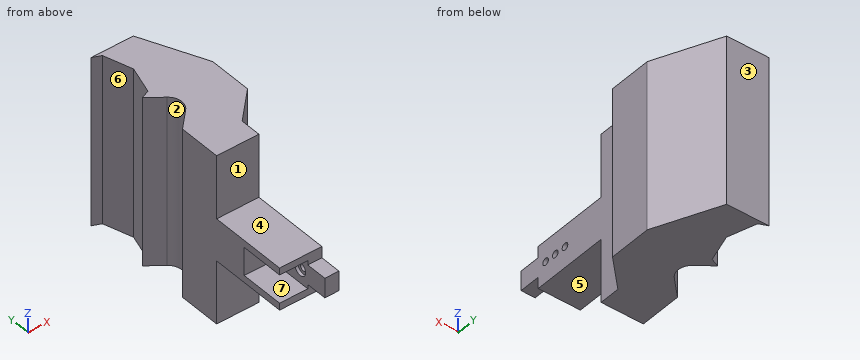
Autodesk Inventor part; units mm, degrees
ref_plane "Work Plane1" through (0, 0, -15) normal (0, 0, 1) x (1, 0, 0)
ref_plane "YZ Plane" through (0, 0, 0) normal (1, 0, 0) x (0, 1, 0)
ref_plane "XZ Plane" through (0, 0, 0) normal (0, 1, 0) x (-1, 0, 0)
sketch "Sketch1" plane through (0, 0, 0) normal (0, 0, 1) x (1, 0, 0)
  line L0 (0, 0) -> (25, 0)
  line L1 (25, 0) -> (25, 40)
  line L2 (25, 40) -> (0, 40)
  line L3 (0, 40) -> (0, 0)
  dimension "d1" = 25
  dimension "d2" = 40
  dimension "d3" = 25
extrude "Extrusion1" add sketch "Sketch1" against normal blind 30
sketch "Sketch2" plane through (25, 0, 0) normal (1, 0, 0) x (0, 0, -1)
  line L0 (0, 0) -> (30, 0)
  circle A0 centre (15, 6.56) radius 2.46
extrude "Extrusion2" cut sketch "Sketch2" against normal blind 30
sketch "Sketch3" plane through (0, 0, 0) normal (-1, 0, 0) x (0, 0, 1)
  line L0 (0, 0) -> (-30, 0)
  line L1 (-25.05, 0) -> (-4.95, 0)
  line L2 (-4.95, 0) -> (-4.95, 33.12)
  line L3 (-4.95, 33.12) -> (-25.05, 33.12)
  line L4 (-25.05, 33.12) -> (-25.05, 0)
  dimension "d11" = 20.1
extrude "Extrusion3" cut sketch "Sketch3" against normal blind 20
sketch "Sketch4" plane through (0, 0, 0) normal (0, -1, 0) x (1, 0, 0)
  line L0 (20, -4.95) -> (20, -25.05)
  line L1 (20, -15) -> (25, -15)
  line L2 (25, 0) -> (25, -30)
  line L3 (20, -8.025) -> (25, -8.025)
  line L4 (25, -8.025) -> (25, -21.975)
  line L5 (25, -21.975) -> (20, -21.975)
  line L6 (20, -21.975) -> (20, -8.025)
  line L7 (20, -8.025) -> (25, -21.975) construction
  line L8 (25, -8.025) -> (20, -21.975) construction
  line L9 (25, -12.54) -> (25, -17.46)
  point P0 (0, 0)
  point P1 (22.5, -15)
  dimension "d14" = 13.95
extrude "Extrusion4" add sketch "Sketch4" along normal blind 15
sketch "Sketch5" plane through (20, 0, 0) normal (-1, 0, 0) x (0, 0, 1)
  circle A0 centre (-15, 6.56) radius 2.46
  circle A1 centre (-15, 6.56) radius 4.7025
  circle A2 centre (-15, 6.56) radius 2.46
  circle A3 centre (-15, 6.56) radius 2.46
  point P0 (0, 0)
  dimension "d17" = 9.405
extrude "Extrusion5" cut sketch "Sketch5" against normal blind 2.1
sketch "Sketch6" plane through (25, 0, 0) normal (1, 0, 0) x (0, 0, -1)
  circle A0 centre (15, 6.56) radius 4.7025
  line L0 (15, 6.56) -> (15, 23.56)
  circle A1 centre (15, 23.56) radius 2.46
  point P0 (0, 0)
  dimension "d20" = 17
  dimension "d21" = 4.92
extrude "Extrusion6" cut sketch "Sketch6" against normal blind 10 contours A1
sketch "Sketch7" plane through (20, 0, 0) normal (-1, 0, 0) x (0, 0, 1)
  circle A0 centre (-15, 23.56) radius 2.46
  circle A1 centre (-15, 23.56) radius 4.7025
  point P0 (0, 0)
  dimension "d24" = 9.405
extrude "Extrusion7" cut sketch "Sketch7" against normal blind 2.1
sketch "Sketch9" plane through (25, 0, 0) normal (1, 0, 0) x (0, 0, -1)
  circle A0 centre (15, 6.56) radius 2.46
  circle A1 centre (15, 6.56) radius 2.46
  circle A2 centre (15, 23.56) radius 2.46
  circle A3 centre (15, 23.56) radius 2.46
  line L0 (30, 40) -> (30, 0)
  line L1 (30, 0) -> (30, 40)
  line L2 (30, 40) -> (0, 40)
  line L3 (0, 40) -> (0, 0)
  line L4 (0, 0) -> (8.025, 0)
  line L5 (21.975, 0) -> (21.975, -15)
  line L6 (21.975, -15) -> (8.025, -15)
  line L7 (8.025, -15) -> (8.025, 0)
  line L8 (0, 0) -> (8.025, 0)
  line L9 (21.975, 0) -> (30, 0)
extrude "Extrusion8" add sketch "Sketch9" along normal blind 5
sketch "Sketch10" plane through (0, 40, 0) normal (0, 1, 0) x (1, 0, 0)
  line L0 (0, 30) -> (30, 30)
  line L1 (30, 0) -> (0, 0)
  line L2 (0, 30) -> (30, 30)
  line L3 (30, 30) -> (30, 0)
  line L4 (30, 0) -> (0, 0)
  line L5 (0, 0) -> (0, 30)
extrude "Extrusion9" add sketch "Sketch10" along normal blind 30
sketch "Sketch12" plane through (30, 0, 0) normal (1, 0, 0) x (0, 0, -1)
  circle A0 centre (15, 6.56) radius 2.46
  line L0 (15, 6.56) -> (15, 15.06)
  circle A1 centre (15, 15.06) radius 2.525
  point P0 (0, 0)
  dimension "d31" = 8.5
  dimension "d33" = 5.05
extrude "Extrusion10" cut sketch "Sketch12" against normal blind 30 contours A1
sketch "Sketch15" plane through (0, 0, -25.05) normal (-1, 0, 0) x (0, 0, 1)
  line L0 (0, 33.12) -> (20.1, 33.12)
  line L1 (20.1, 33.12) -> (20.1, 0)
  line L2 (0, 33.12) -> (20.1, 33.12)
  line L3 (20.1, 33.12) -> (20.1, 31.1)
  line L4 (20.1, 31.1) -> (0, 31.1)
  line L5 (0, 31.1) -> (0, 33.12)
  point P0 (25.05, 0)
  dimension "d57" = 2.02
extrude "Extrusion13" add sketch "Sketch15" against normal blind 20
sketch "Sketch17" plane through (0, 0, 0) normal (0, 0, 1) x (1, 0, 0)
  line L0 (0, 70) -> (30, 70)
  line L1 (30, 70) -> (50.0622, 90.0622)
  line L2 (30, 70) -> (80, 70) construction
  line L3 (11.9522, 97.2454) -> (0, 85.2932)
  line L4 (0, 70) -> (0, 85.2932)
  line L5 (0, 70) -> (0, 0)
  line L6 (0, 70) -> (30, 70)
  line L7 (10.923, 112.2849) -> (0, 120.567)
  line L8 (50.0622, 105.3553) -> (50.0622, 120.567)
  line L9 (50.0622, 105.3553) -> (50.0622, 90.0622)
  arc A0 (11.9522, 97.2454) -> (10.923, 112.2849) centre (4.8811, 104.3165) ccw
  line L10 (0, 165.567) -> (30, 165.567)
  line L11 (30, 165.567) -> (50.0622, 120.567)
  line L12 (6, 163.067) -> (0, 165.567)
  line L13 (6, 123.067) -> (0, 120.567)
  line L14 (6, 123.067) -> (12, 143.067)
  line L15 (12, 143.067) -> (6, 163.067)
  dimension "d61" = 45
  dimension "d62" = 32.0271
  dimension "d72" = 10
extrude "Extrusion14" add sketch "Sketch17" against normal blind 30
sketch "Sketch24" plane through (0, 0, 0) normal (0, 0, 1) x (1, 0, 0)
  line L0 (30, 70) -> (50.0622, 90.0622)
  line L1 (30, 70) -> (50.0622, 90.0622)
  line L2 (50.0622, 90.0622) -> (50.0622, 120.567)
  line L3 (50.0622, 90.0622) -> (50.0622, 120.567)
  line L4 (30, 165.567) -> (50.0622, 120.567)
  line L5 (50.0622, 120.567) -> (30, 165.567)
  line L6 (0, 165.567) -> (30, 165.567)
  line L7 (30, 165.567) -> (0, 165.567)
  line L8 (6, 163.067) -> (0, 165.567)
  line L9 (0, 165.567) -> (6, 163.067)
  line L10 (12, 143.067) -> (6, 163.067)
  line L11 (6, 163.067) -> (12, 143.067)
  line L12 (6, 123.067) -> (12, 143.067)
  line L13 (12, 143.067) -> (6, 123.067)
  line L14 (0, 120.567) -> (6, 123.067)
  line L15 (6, 123.067) -> (0, 120.567)
  line L16 (10.923, 112.2849) -> (0, 120.567)
  line L17 (0, 120.567) -> (10.923, 112.2849)
  line L18 (0, 85.2932) -> (11.9522, 97.2454)
  line L19 (11.9522, 97.2454) -> (0, 85.2932)
  line L20 (0, 85.2932) -> (0, 55.2932)
  line L21 (0, 0) -> (0, 85.2932)
  line L22 (0, 55.2932) -> (30, 55.2932)
  line L23 (30, 0) -> (30, 70)
  line L24 (30, 55.2932) -> (30, 70)
  arc A0 (11.9522, 97.2454) -> (10.923, 112.2849) centre (4.8811, 104.3165) ccw
  arc A1 (11.9522, 97.2454) -> (10.923, 112.2849) centre (4.8811, 104.3165) ccw
  dimension "d102" = 30
extrude "Extrusion15" add sketch "Sketch24" along normal blind 45
ref_plane "Work Plane1" through (0, 0, -15) normal (0, 0, 1) x (1, 0, 0)
mirror "Mirror1" about plane through (0, 0, -15) normal (0, 0, 1) of "Extrusion15"
properties part number "rec_c_40mm_x_120mm"
Could you check a few things on this model? Use its own coordinates, in mm. Face numbers are marked on the shaded views. A direction names the side the tool comes from. Coordinates: 2 decimals unless noted, no trailing zeros. Write each loop counter-clockwise with the first axis right and the second up, starting at its lowest first coordinate (ties: lowest second). Pieces come first, ordered by that corner, then holes. Notation, with made-up numbers: M -22,1.25 L 17,1.25 A34 cw 17,32.25 Z; hole C 63,66.25 d3. An arc over 180 degrees is marked long. Answer as CSV lines item,"result". Start each with the question number.
1) I want a section at C-C, the plane z = -47. Please give me the cut outline in (x, y), and give its area (3 significant figures).
2) For P1, Ø4.5, axis at y = 21.5, z = -13.5, coming from the -X side; P2, Ø9, axis at x = 10.5, z = -5.5, coming from the -Y side; P3, Ø16, axis at x = 12.5, y = 18.5, coming from the +Z side; P4, Ø3, axis at y = 6.56, z = -15, coming from the -X side (1 decimal), each with a flat end and sliding along its axis, tell me the tip position at first contact or that it passes through.
3) Please list where these lines run through material, in increasing order: line 1 (Y direction, x = 27.75, z = -15) (3 decimals); line 2 (Z direction, x = 24.5, y = 6.56); line 3 (Y direction, x = 21, z = -15) (1 decimal). Write a range as from..to.
4) I want a section at A-A, the plane y = 15.06. Please give me the cut outline in (x, z) (3 decimals), and give its area (4 significant figures).
5) For the marked faces 5, 6 and 7, which set-ups out of +Z, -Z, +X, -X, +Y, -Y let a thin tool reach every point of the face, with its end or its side?
6) We'd pull the mould along Y, two halves only. Please class the marked faces 1, 2, 3 and 4: +Y half, -Y half, draft (parallel to the pull), parting line (faces both ways), or undercut.
7) I want a section at D-D, the plane z = -15. Give the number of separate pieces and of enclosed holes in the cut face, and give its area (3 significant figures).
8) I want a section at B-B, the plane x = 9. Please give me the cut outline in (y, z), and give its area (3 significant figures).
Data:
1,outline,"M 0,55.29 L 30,55.29 L 30,70 L 50.06,90.06 L 50.06,120.57 L 30,165.57 L 0,165.57 L 6,163.07 L 12,143.07 L 6,123.07 L 0,120.57 L 10.92,112.28 A10 cw 11.95,97.25 L 0,85.29 Z"
1,area,"3,870 mm^2"
2,P1,"stops at x = 20"
2,P2,"stops at y = 0"
2,P3,"stops at z = 0"
2,P4,"passes through"
3,line 1,"y = -15..4.1, 9.02..12.535, 17.585..21.1, 26.02..165.567"
3,line 2,"z = -30..-17.46, -12.54..0"
3,line 3,"y = -15..1.9, 11.3..12.5, 17.6..18.9, 28.3..165.6"
4,outline,"M 0,-30 L 30,-30 L 30,-17.525 L 20,-17.525 L 20,-25.05 L 0,-25.05 Z; M 0,-4.95 L 20,-4.95 L 20,-12.475 L 30,-12.475 L 30,0 L 0,0 Z"
4,area,"447.5 mm^2"
5,face 5,"-Z, +X, -X, -Y"
5,face 6,"+Z, -Z, -X"
5,face 7,"-X, -Y"
6,face 1,"-Y half"
6,face 2,"undercut"
6,face 3,"+Y half"
6,face 4,"draft"
7,separate pieces,"4"
7,enclosed holes,"0"
7,area,"4,890 mm^2"
8,outline,"M 0,-30 L 55.29,-30 L 55.29,-75 L 94.29,-75 L 94.29,45 L 55.29,45 L 55.29,0 L 0,0 L 0,-4.95 L 31.1,-4.95 L 31.1,-25.05 L 0,-25.05 Z; M 113.74,-75 L 133.07,-75 L 133.07,45 L 113.74,45 Z; M 153.07,-75 L 165.57,-75 L 165.57,45 L 153.07,45 Z"
8,area,"9,530 mm^2"
